Input: part model. Units: mm. Frame: model coordinates. Face numbers are marked on the shaded views. A direction names the side the tool comes from. Give positions to 0.01 mm unless a question says otherwise; leave off trailing zeros. Loops run counter-clockwise (first coordinate to the right, second up) from the corner with the lowest first, then second, coordinate; pieces in that order, holes last. Notation, with made-up numbers: M -25.75,15 L -2.75,15 A31 ccw -2.75,51 Z; hole C 56,-28 d9. An arc over 180 degrees is marked long. One line per item, written item: value. Start each with the question number.
(1) Pull-direction query (Z, two-part tool) for the marked faces 4, 5 and 6; classes: released by +Z, released by -Z, zero draft, split by the parting line, or undercut.
(2) Pin query (flat end, axial travel): P1, Ø7, axis at x = 20, z = 10, coming from the -Y side; P2, Ø1.9, axis at x = 20, z = 10, coming from the +Y side; P3, Ø4, axis at x = 20, z = -10, coming from the +Y side. Return the tip coordinate at first contact, or that it passes through.
(3) Section B-B on x = 0.5. Output: boundary loops of the cut face in (y, z).
(4) Section C-C on y = 2.1. Output: boundary loops of the cut face in (x, z).
(5) Section D-D on x = 21. Output: boundary loops of the cut face in (y, z), plus the area to 3 significant figures.
(6) Access query for the marked faces 1, 2 and 3. Directions: +Z, -Z, +X, -X, +Y, -Y. A direction counts if a zero-diameter tool reaches every point of the face in a straight line with its end or side. Return the directions, or none.
(7) Ray query, line 1 along X through (y, z) = (4.25, -10) (3 decimals); line 2 along Z through (x, y) = (20, 3.85) (3 decimals); line 3 along X through (y, z) = (1.2, 10). Return the intervals inside material, ascending. Write a range as from..to.
(8) Section A-A on z = 3.75. Output: boundary loops of the cut face in (x, y).
```python
from build123d import *

# Parameters (mm, degrees)
SKETCH1_W           = 50
SKETCH1_H           = 30
SKETCH1_R           = 1.55
BOSS_EXTRUDE1_DEPTH = 5
SKETCH2_R           = 2.625
CUT_EXTRUDE1_DEPTH  = 2
SKETCH3_W           = 31.5
SKETCH3_H           = 13
CUT_EXTRUDE2_DEPTH  = 1.2
FILLET1_R           = 5


with BuildPart() as part:
    # Sketch1 → Boss-Extrude1 (new body)
    with BuildSketch(Plane(origin=(0, 0, 0), x_dir=(1, 0, 0), z_dir=(0, 1, 0))):
        Rectangle(SKETCH1_W, SKETCH1_H)
        with Locations((-20, -10)):
            Circle(SKETCH1_R, mode=Mode.SUBTRACT)
        with Locations((20, -10)):
            Circle(SKETCH1_R, mode=Mode.SUBTRACT)
        with BuildLine():
            Line((7, -5), (-11, -5))
            Line((-11, -5), (-11, -3.25))
            Line((-11, -3.25), (-14.5, -3.25))
            ThreePointArc((-14.5, -3.25), (-17.75, 0), (-14.5, 3.25))
            Line((-14.5, 3.25), (-11, 3.25))
            Line((-11, 3.25), (-11, 5))
            Line((-11, 5), (7, 5))
            Line((7, 5), (7, 3.25))
            Line((7, 3.25), (10.5, 3.25))
            ThreePointArc((10.5, 3.25), (12.798097039, 2.298097039), (13.75, 0))
            ThreePointArc((13.75, 0), (12.798097039, -2.298097039), (10.5, -3.25))
            Line((10.5, -3.25), (7, -3.25))
            Line((7, -3.25), (7, -5))
        make_face(mode=Mode.SUBTRACT)
        with Locations((-20, 10)):
            Circle(SKETCH1_R, mode=Mode.SUBTRACT)
        with Locations((20, 10)):
            Circle(SKETCH1_R, mode=Mode.SUBTRACT)
    extrude(amount=BOSS_EXTRUDE1_DEPTH)

    # Sketch2 → Cut-Extrude1 (cut)
    with BuildSketch(Plane(origin=(0, 5, 0), x_dir=(1, 0, 0), z_dir=(0, 1, 0))):
        with Locations((-20, 10)):
            Circle(SKETCH2_R)
        with Locations((20, 10)):
            Circle(SKETCH2_R)
        with Locations((20, -10)):
            Circle(SKETCH2_R)
        with Locations((-20, -10)):
            Circle(SKETCH2_R)
    extrude(amount=-CUT_EXTRUDE1_DEPTH, mode=Mode.SUBTRACT)

    # Sketch3 → Cut-Extrude2 (cut)
    with BuildSketch(Plane.XZ):
        with Locations((-2, 0)):
            Rectangle(SKETCH3_W, SKETCH3_H)
    extrude(amount=-CUT_EXTRUDE2_DEPTH, mode=Mode.SUBTRACT)

    # Fillet1
    fillet1_edges = [part.edges().sort_by_distance(p)[0] for p in [
        (-25, 2.5, 15),
        (-25, 2.5, -15),
        (25, 2.5, -15),
        (25, 2.5, 15),
    ]]
    fillet(fillet1_edges, radius=FILLET1_R)


solid = part.part
```
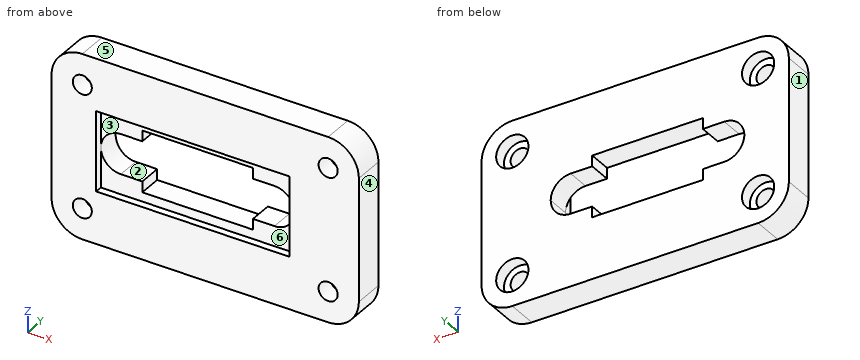
Output values:
1. face 4: zero draft
1. face 5: released by +Z
1. face 6: undercut
2. P1: stops at y = 0
2. P2: passes through
2. P3: stops at y = 3
3. outline: M 0,-15 L 5,-15 L 5,-5 L 1.2,-5 L 1.2,-6.5 L 0,-6.5 Z; M 0,6.5 L 1.2,6.5 L 1.2,5 L 5,5 L 5,15 L 0,15 Z
4. outline: M -25,-10 A5 ccw -20,-15 L 20,-15 A5 ccw 25,-10 L 25,10 A5 ccw 20,15 L -20,15 A5 ccw -25,10 Z; hole C -20,-10 d3.1; hole C -20,10 d3.1; hole M -14.5,-3.25 L -11,-3.25 L -11,-5 L 7,-5 L 7,-3.25 L 10.5,-3.25 A3.25 ccw 10.5,3.25 L 7,3.25 L 7,5 L -11,5 L -11,3.25 L -14.5,3.25 A3.25 ccw Z; hole C 20,-10 d3.1; hole C 20,10 d3.1
5. outline: M 0,-14.9 L 5,-14.9 L 5,-12.43 L 3,-12.43 L 3,-11.18 L 0,-11.18 Z; M 0,-8.82 L 3,-8.82 L 3,-7.57 L 5,-7.57 L 5,7.57 L 3,7.57 L 3,8.82 L 0,8.82 Z; M 0,11.18 L 3,11.18 L 3,12.43 L 5,12.43 L 5,14.9 L 0,14.9 Z
5. area: 115 mm²
6. face 1: +Z, -Z, -X, +Y, -Y
6. face 2: +Y, -Y
6. face 3: -Y
7. line 1: x = -25..-22.625, -17.375..17.375, 22.625..25
7. line 2: z = -15..-12.625, -7.375..7.375, 12.625..15
7. line 3: x = -25..-21.55, -18.45..18.45, 21.55..25
8. outline: M -25,0 L -17.75,0 L -17.75,1.2 L -11,1.2 L -11,5 L -25,5 Z; M 7,1.2 L 13.75,1.2 L 13.75,0 L 25,0 L 25,5 L 7,5 Z
